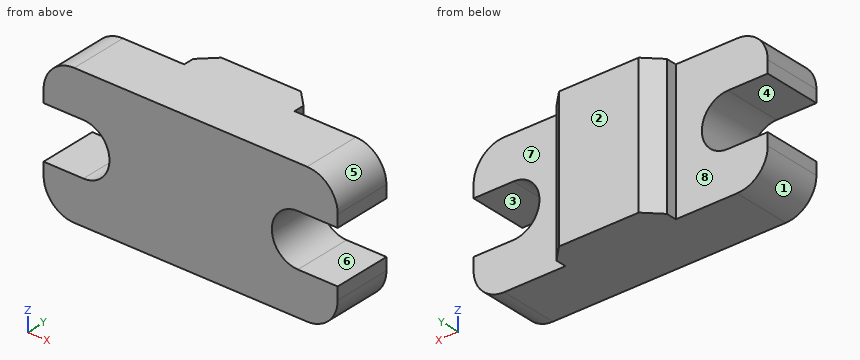
```python
from build123d import *

# Parameters (mm, degrees)
BOSS_EXTRUDE1_DEPTH = 3.8
SKETCH3_W           = 7.2
SKETCH3_H           = 9
BOSS_EXTRUDE2_DEPTH = 1.7
CHAMFER1_SIZE       = 1


with BuildPart() as part:
    # Sketch1 → Boss-Extrude1 (new body)
    with BuildSketch(Plane(origin=(0, 0, 0), x_dir=(1, 0, 0), z_dir=(0, 1, 0))):
        with BuildLine():
            Line((0, 6.2), (2.6, 6.2))
            ThreePointArc((2.6, 6.2), (4.3, 4.5), (2.6, 2.8))
            Line((2.6, 2.8), (0, 2.8))
            Line((0, 2.8), (0, 2))
            ThreePointArc((0, 2), (0.585786438, 0.585786438), (2, 0))
            Line((2, 0), (17.2, 0))
            ThreePointArc((17.2, 0), (18.614213562, 0.585786438), (19.2, 2))
            Line((19.2, 2), (19.2, 2.8))
            Line((19.2, 2.8), (16.6, 2.8))
            ThreePointArc((16.6, 2.8), (14.9, 4.5), (16.6, 6.2))
            Line((16.6, 6.2), (19.2, 6.2))
            Line((19.2, 6.2), (19.2, 7))
            ThreePointArc((19.2, 7), (18.614213562, 8.414213562), (17.2, 9))
            Line((17.2, 9), (2, 9))
            ThreePointArc((2, 9), (0.585786438, 8.414213562), (0, 7))
            Line((0, 7), (0, 6.2))
        make_face()
    extrude(amount=BOSS_EXTRUDE1_DEPTH)

    # Sketch3 → Boss-Extrude2 (add)
    with BuildSketch(Plane(origin=(0, 3.8, 0), x_dir=(1, 0, 0), z_dir=(0, 1, 0))):
        with Locations((9.6, 4.5)):
            Rectangle(SKETCH3_W, SKETCH3_H)
    extrude(amount=BOSS_EXTRUDE2_DEPTH)

    # Chamfer1
    chamfer1_edges = [part.edges().sort_by_distance(p)[0] for p in [
        (13.2, 5.5, -4.5),
        (6, 5.5, -4.5),
    ]]
    chamfer(chamfer1_edges, length=CHAMFER1_SIZE)


solid = part.part
```
Verification items for the finished model (mm, model axes). Face numbers are marked on the shaded views. A direction names the side the tool comes from. Give positions to 0.01 mm unless a question says otherwise; leave off trailing zeros. Loops run counter-clockwise (first coordinate to the right, second up) from the corner with the lowest first, then second, coordinate; pieces in that order, holes last. Notation, with made-up numbers: M 83.5,15 L 139.5,15 A25 ccw 139.5,39 Z; hole C 65,21.5 d8. An arc over 180 degrees is marked long. Return JSON: item names as keys, results as strings.
1) Section check B-B, the plane y = 1.1. Enter the section's corners in (x, z).
Findings:
{"outline": "M 0,-7 A2 ccw 2,-9 L 17.2,-9 A2 ccw 19.2,-7 L 19.2,-6.2 L 16.6,-6.2 A1.7 cw 16.6,-2.8 L 19.2,-2.8 L 19.2,-2 A2 ccw 17.2,0 L 2,0 A2 ccw 0,-2 L 0,-2.8 L 2.6,-2.8 A1.7 cw 2.6,-6.2 L 0,-6.2 Z"}
2) Tool access check on the marked faces 4, 5, 6, 7 and 8. Record the directions out of +Z, -Z, +X, -X, +Y, -Y that give a thin tool (end or side, any length) a straight path to the whole face; none if there is none.
Findings:
{"face 4": "-X, +Y, -Y", "face 5": "+Z, +X, +Y, -Y", "face 6": "+X, +Y, -Y", "face 7": "+Z, -Z, +X, +Y", "face 8": "+Z, -Z, -X, +Y"}
3) Mould release check, pull along Z, two halves, no side actions. Record for the marked faces 1, 2 and 3: released by +Z, released by -Z, zero draft, split by the parting line, or undercut.
Findings:
{"face 1": "released by -Z", "face 2": "zero draft", "face 3": "undercut"}
4) Gauge pin test, flat ends, axial feed: P1, Ø1, axis at y = 1, z = -4, coming from the +X side; P2, Ø3, axis at y = 4.5, z = -2, coming from the +X side; P3, Ø1.5, axis at y = 1.5, z = -5, coming from the +X side; P4, Ø0.8, axis at x = 1, y = 1, coming from the -Z side. Record the tip position at first contact, or that the pin passes through.
Findings:
{"P1": "stops at x = 15.23", "P2": "stops at x = 19.2", "P3": "stops at x = 15.45", "P4": "stops at z = -8.91"}
5) Section check A-A, the plane z = -4.5. Enter the section's corners in (x, y).
Findings:
{"outline": "M 4.3,0 L 14.9,0 L 14.9,3.8 L 13.2,3.8 L 13.2,4.5 L 12.2,5.5 L 7,5.5 L 6,4.5 L 6,3.8 L 4.3,3.8 Z"}
6) Material ranges on L1, parallel to Y at x = 4.5, z = -2.5; L2, parallel to X at y = 4.25, z = -2.25; L3, parallel to Y at x = 12.25, z = -7, recorded low to high. Write a range as [from, to].
Findings:
{"L1": "y = [0, 3.8]", "L2": "x = [6, 13.2]", "L3": "y = [0, 5.45]"}
7) Section check C-C, the plane y = 4.95. Enter the section's corners in (x, z).
Findings:
{"outline": "M 6.45,-9 L 12.75,-9 L 12.75,0 L 6.45,0 Z"}
8) Section check D-D, the plane z = -7.25. Enter the section's corners in (x, y).
Findings:
{"outline": "M 0.02,0 L 19.18,0 L 19.18,3.8 L 13.2,3.8 L 13.2,4.5 L 12.2,5.5 L 7,5.5 L 6,4.5 L 6,3.8 L 0.02,3.8 Z"}
